```python
from build123d import *

# Parameters (mm, degrees)
F1_R     = 24.1613499239
F2_DEPTH = 4
F0_W     = 76.2569829822
F0_H     = 79.4832408428
F3_DEPTH = 1
F4_R     = 2.0739165502
F5_DEPTH = 1
F6_R     = 2.8886313869
F6_R_2   = 2.3646284302
F6_R_3   = 2.1352299697
F7_DEPTH = 1


# Not quite as in the source:
# - a fillet or chamfer that OpenCascade refuses, or shapes differently, is made with other operations: its cross-section is extruded or revolved along the edge and cut away or added


with BuildPart() as f2:
    # F1 (on face) → F2 (new body)
    with BuildSketch(Plane.XY):
        Circle(F1_R)
    extrude(amount=F2_DEPTH)

    # F0 (on Top) → F3 (join)
    with BuildSketch(Plane.XY):
        Rectangle(F0_W, F0_H)
    extrude(amount=F3_DEPTH)

    # F4 (on face) → F5 (join)
    with BuildSketch(Plane.XY.offset(1)):
        with Locations((-27.2765364498, -30.6494422257)):
            Circle(F4_R)
    extrude(amount=F5_DEPTH)

    # F6 (on face) → F7 (join)
    with BuildSketch(Plane.XY.offset(1)):
        with Locations((27.8631281108, -30.0628505647)):
            Circle(F6_R)
        with Locations((27.8631281108, 30.6494422257)):
            Circle(F6_R_2)
        with Locations((-27.8631299734, 30.6494422257)):
            Circle(F6_R_3)
    extrude(amount=F7_DEPTH)

    # F8: chamfer of 10 on 1 edges, made by hand


with BuildPart() as f8_tool2:
    # F8_s3 → F8_t4 (revolve)
    with BuildSketch(Plane.XZ):
        with BuildLine():
            Line((24.4441926363, -6.2828427125), (13.8785072114, 4.2828427125))
            Line((13.8785072114, 4.2828427125), (13.8785072114, 4.4828427125))
            ThreePointArc((13.8785072114, 4.4828427125), (19.0199285676, 4.2), (24.1613499239, 4.2))
            Line((24.1613499239, 4.2), (24.3613499239, 4))
            ThreePointArc((24.3613499239, 4), (24.3613499239, -1.1414213562), (24.6441926363, -6.2828427125))
            Line((24.6441926363, -6.2828427125), (24.4441926363, -6.2828427125))
        make_face()
    revolve(axis=Axis((0, 0, 4), (0, 0, 1)))

    split(bisect_by=Plane.XY.offset(1), keep=Keep.TOP)


with BuildPart() as f2_1:
    add(f2.part)

    # F8_t1: cut F8_tool2
    add(f8_tool2.part, mode=Mode.SUBTRACT)


solid = f2_1.part
```
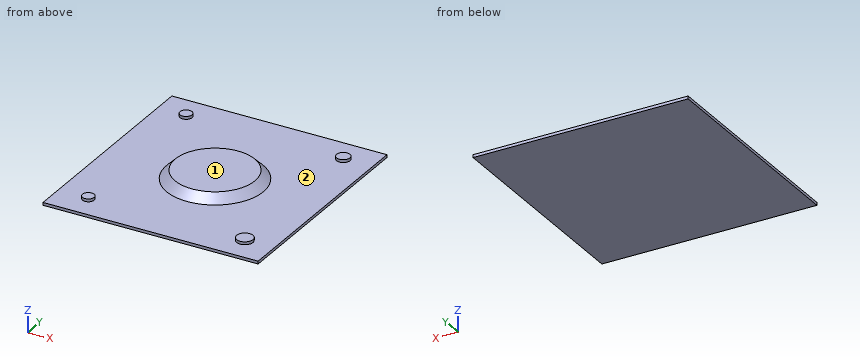
Model file for the job. Use its own axes, mm. Face numbers are marked on the shaded views. A direction names the side the tool comes from. Give positions to 0.01 mm unless a question says otherwise; leave off trailing zeros. Write each loop counter-clockwise with the first axis right and the second up, starting at its lowest first coordinate (ties: lowest second). Pieces come first, ordered by that corner, then holes. Notation, with made-up numbers: M 88,-23.75 L 103,-23.75 A28 ccw 103,6.25 Z; hole C -19.5,0 d9. An arc over 180 degrees is marked long. Use a Markdown table: item, result.
1) Cut at A-A (y = 0). List the corners of the cut face in (x, z), and give its area (3 significant figures).
Responses:
| item | result |
|---|---|
| outline | M -38.13,0 L 38.13,0 L 38.13,1 L 17.16,1 L 14.16,4 L -14.16,4 L -17.16,1 L -38.13,1 Z |
| area | 170 mm2 |
2) Pin check, flat tips, straight feed: pin 1 (1.2 mm diameter, centred on x = -27, y = -30, fed in from +Z); pin 2 (8 mm diameter, centred on x = 19, y = -14, fed in from -Z); pin 3 (12 mm diameter, centred on x = 17, y = 30, fed in from +Z). Stop position of each tip, or through.
Responses:
| item | result |
|---|---|
| pin 1 | stops at z = 2 |
| pin 2 | stops at z = 0 |
| pin 3 | stops at z = 1 |
3) Drill centre lines: line 1 (X direction, y = 30.5, z = 1.75); line 2 (Z direction, x = -18.5, y = -22.5); line 3 (Y direction, x = -6, z = 2.35). Where is each one in solid material? Low to high. Write a range as from..to.
Responses:
| item | result |
|---|---|
| line 1 | x = -29.99..-25.73, 25.5..30.22 |
| line 2 | z = 0..1 |
| line 3 | y = -14.63..14.63 |
4) Tool access for the marked faces 1 and 2: list every direction of +Z, -Z, +X, -X, +Y, -Y with a clear straight run to the whole face (end or side of a thin tool).
Responses:
| item | result |
|---|---|
| face 1 | +Z, +X, -X, +Y, -Y |
| face 2 | +Z |
5) Cut at C-C (z = 3). List the corners of the cut face in (x, y).
Responses:
| item | result |
|---|---|
| outline | C 0,0 d30.32 |
6) Cut at D-D (y = -19.5). List the corners of the cut face in (x, z).
Responses:
| item | result |
|---|---|
| outline | M -38.13,0 L 38.13,0 L 38.13,1 L -38.13,1 Z |
7) Cut at B-B (x = 0). List the corners of the cut face in (y, z).
Responses:
| item | result |
|---|---|
| outline | M -39.74,0 L 39.74,0 L 39.74,1 L 17.16,1 L 14.16,4 L -14.16,4 L -17.16,1 L -39.74,1 Z |
